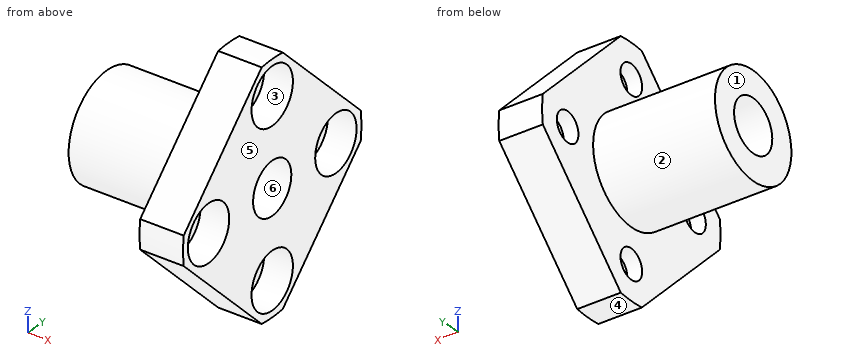
```python
from build123d import *

# Parameters (mm, degrees)
BOSS_EXTRUDE1_DEPTH                              = 5
SKETCH2_W                                        = 14
SKETCH2_H                                        = 6
F_6_0_6_DIAMETER_HOLE1_D                         = 6
F_6_0_6_DIAMETER_HOLE1_DEPTH                     = 19
CBORE_FOR_M3_HEX_HEAD_MACHINE_SCREW1_D           = 3.4
CBORE_FOR_M3_HEX_HEAD_MACHINE_SCREW1_DEPTH       = 19
CBORE_FOR_M3_HEX_HEAD_MACHINE_SCREW1_CBORE_D     = 6.5
CBORE_FOR_M3_HEX_HEAD_MACHINE_SCREW1_CBORE_DEPTH = 3.3


with BuildPart() as part:
    # Sketch1 → Boss-Extrude1 (new body)
    with BuildSketch(Plane(origin=(14, 0, 0), x_dir=(0, -1, 0), z_dir=(-1, 0, 0))):
        with BuildLine():
            Line((-1.654450236, 13.90189895), (-13.90189895, 1.654450236))
            ThreePointArc((-13.90189895, 1.654450236), (-14, 0), (-13.90189895, -1.654450236))
            Line((-13.90189895, -1.654450236), (-1.654450236, -13.90189895))
            ThreePointArc((-1.654450236, -13.90189895), (0, -14), (1.654450236, -13.90189895))
            Line((1.654450236, -13.90189895), (13.90189895, -1.654450236))
            ThreePointArc((13.90189895, -1.654450236), (14, 0), (13.90189895, 1.654450236))
            Line((13.90189895, 1.654450236), (1.654450236, 13.90189895))
            ThreePointArc((1.654450236, 13.90189895), (0, 14), (-1.654450236, 13.90189895))
        make_face()
    extrude(amount=-BOSS_EXTRUDE1_DEPTH)

    # Sketch2 → Revolve1 (revolve)
    with BuildSketch(Plane(origin=(0, 0, 0), x_dir=(-1, 0, 0), z_dir=(0, 0, -1))):
        with Locations((-7, 3)):
            Rectangle(SKETCH2_W, SKETCH2_H)
    revolve(axis=Axis((14, 0, 0), (-1, 0, 0)))

    # Ø6.0 (6) Diameter Hole1
    with Locations(Plane(origin=(19, 0, 0), x_dir=(0, 0, -1), z_dir=(1, 0, 0))):
        with Locations((0, 0)):
            Hole(F_6_0_6_DIAMETER_HOLE1_D / 2, depth=F_6_0_6_DIAMETER_HOLE1_DEPTH)

    # CBORE for M3 Hex Head Machine Screw1
    with Locations(Plane(origin=(19, 0, 0), x_dir=(0, 0, -1), z_dir=(1, 0, 0))):
        with Locations((0, -10), (10, 0), (-10, 0), (0, 10)):
            CounterBoreHole(CBORE_FOR_M3_HEX_HEAD_MACHINE_SCREW1_D / 2, CBORE_FOR_M3_HEX_HEAD_MACHINE_SCREW1_CBORE_D / 2, CBORE_FOR_M3_HEX_HEAD_MACHINE_SCREW1_CBORE_DEPTH, depth=CBORE_FOR_M3_HEX_HEAD_MACHINE_SCREW1_DEPTH)


solid = part.part
```
Verification items for the finished model (mm, model axes). Face numbers are marked on the shaded views. A direction names the side the tool comes from. Give positions to 0.01 mm unless a question says otherwise; leave off trailing zeros. Loops run counter-clockwise (first coordinate to the right, second up) from the corner with the lowest first, then second, coordinate; pieces in that order, holes last.
1. Section check A-A, the plane z = 0. Enter the section's corners in (x, y), then the cut area to 3 significant figures.
2. Section check C-C, the plane z = -10. Enter the section's corners in (x, y), then the cut area to 3 significant figures.
3. Go/stop test with flat-tipped pins: pin 1 Ø3 at (y, z) = (10.5, 0.5) entering from +X; pin 2 Ø5.5 at (y, z) = (0, -10) entering from -X; pin 3 Ø1 at (x, z) = (10.5, 6) entering from +Y; pin 4 Ø2 at (y, z) = (10, 0) entering from +X. Record where each tip stops, or that it passes through.
4. Section check D-D, the plane x = 4.5. Enter the section's corners in (y, z).
5. Set-up check for the marked faces 1, 2 and 3: record each of +Z, -Z, +X, -X, +Y, -Y from which the full face is reachable in a straight line by a thin tool's end or side.
6. Mould release check, pull along Y, two halves, no side actions. Record for the marked faces 4, 5 and 6: released by +Y, released by -Y, zero draft, split by the parting line, or undercut.
7. Thickness scan on line 1 (Y direction, x = 14.7, z = 0); line 2 (Y direction, x = 17.05, z = 0); line 3 (Y direction, x = 4.75, z = 0). Record the ranges inside material, lowest first.
Geometry says:
1. outline: (0, -6) - (14, -6) - (14, -8.3) - (15.7, -8.3) - (15.7, -6.75) - (19, -6.75) - (19, -3) - (0, -3) - close; (0, 3) - (19, 3) - (19, 6.75) - (15.7, 6.75) - (15.7, 8.3) - (14, 8.3) - (14, 6) - (0, 6) - close; (14, -14) - (19, -14) - (19, -13.25) - (15.7, -13.25) - (15.7, -11.7) - (14, -11.7) - close; (14, 11.7) - (15.7, 11.7) - (15.7, 13.25) - (19, 13.25) - (19, 14) - (14, 14) - close
1. area: 140 mm2
2. outline: (14, -5.56) - (19, -5.56) - (19, -3.25) - (15.7, -3.25) - (15.7, -1.7) - (14, -1.7) - close; (14, 1.7) - (15.7, 1.7) - (15.7, 3.25) - (19, 3.25) - (19, 5.56) - (14, 5.56) - close
2. area: 28.3 mm2
3. pin 1: stops at x = 15.7
3. pin 2: stops at x = 14
3. pin 3: stops at y = 2.4
3. pin 4: passes through
4. outline: circle Ø12 at (0, 0); hole circle Ø6 at (0, 0)
5. face 1: +Z, -Z, -X, +Y, -Y
5. face 2: -X
5. face 3: +X
6. face 4: split by the parting line
6. face 5: zero draft
6. face 6: undercut
7. line 1: y = -14 to -11.7, -8.3 to -3, 3 to 8.3, 11.7 to 14
7. line 2: y = -14 to -13.25, -6.75 to -3, 3 to 6.75, 13.25 to 14
7. line 3: y = -6 to -3, 3 to 6
